Geometry: final body of the model. Coordinates: model frame, mm. Face numbers are marked on the shaded views. A direction names the side the tool comes from. Coordinates: 2 decimals unless noted, no trailing zeros. Order: outer loops, then holes, each group sorted by start corner. A loop starts at its lowest first (then second) coordinate and runs counter-clockwise, first axis right, second up. Notation, with made-up numbers: (-34.75, 88.5) -> (5.25, 88.5) arc R22 cw to (5.25, 111.5) -> close; hole circle Ø8 at (37.25, -21.5). An arc over 180 degrees is marked (long way). Use one line per item in the form item = value.
```python
from build123d import *

# Parameters (mm, degrees)
SKIZZE1_W                       = 36
SKIZZE1_H                       = 38
AUFSATZ_LINEAR_AUSTRAGEN2_DEPTH = 40
VERRUNDUNG1_R                   = 1
SCHNITT_LINEAR_AUSTRAGEN1_REACH = 74.681
SKIZZE2_W                       = 30
SKIZZE2_H                       = 30
VERRUNDUNG2_R                   = 6
DURCHGANGSLOCH_F_R_M31_D        = 3.4
DURCHGANGSLOCH_F_R_M31_DEPTH    = 3
DURCHGANGSLOCH_F_R_M31_TIP      = 1.021463052
SKIZZE5_W                       = 2.5
SKIZZE5_H                       = 38
SKIZZE5_W_2                     = 1
AUFSATZ_LINEAR_AUSTRAGEN3_DEPTH = 2
SKIZZE8_W                       = 1
SKIZZE8_H                       = 38
SCHNITT_LINEAR_AUSTRAGEN3_DEPTH = 1
SKIZZE6_W                       = 2.5
SKIZZE6_H                       = 38
SKIZZE6_W_2                     = 1
AUFSATZ_LINEAR_AUSTRAGEN4_DEPTH = 2
SKIZZE9_W                       = 1
SKIZZE9_H                       = 38
SCHNITT_LINEAR_AUSTRAGEN4_DEPTH = 1
VERRUNDUNG3_R                   = 1
VERRUNDUNG4_R                   = 1
SCHNITT_LINEAR_AUSTRAGEN2_REACH = 75.338
VERRUNDUNG9_R                   = 1
VERRUNDUNG10_R                  = 10


with BuildPart() as part:
    # Skizze1 → Aufsatz-Linear austragen2 (new body)
    with BuildSketch(Plane(origin=(0, 0, 0), x_dir=(1, 0, 0), z_dir=(0, 1, 0))):
        with BuildLine():
            Line((20, -21), (20, 21))
            ThreePointArc((20, 21), (19.460793496, 22.319706051), (18.151722222, 22.884241359))
            ThreePointArc((18.151722222, 22.884241359), (7.231561818, 25.331524584), (-1.857986079, 31.859864147))
            Line((-1.857986079, 31.859864147), (-27.041617117, 22.693772058))
            ThreePointArc((-27.041617117, 22.693772058), (-31.15076398, 18.70575902), (-30.908104914, 12.984705575))
            ThreePointArc((-30.908104914, 12.984705575), (-27.294602816, 1.09378988), (-27.822222222, -11.322847799))
            ThreePointArc((-27.822222222, -11.322847799), (-26.22162429, -18.029054702), (-20, -21))
            Line((-20, -21), (20, -21))
        make_face()
        Rectangle(SKIZZE1_W, SKIZZE1_H, mode=Mode.SUBTRACT)
        with BuildLine():
            Line((16, 21), (-20, 21))
            Line((-20, 21), (-20, -18))
            ThreePointArc((-20, -18), (-23.888515181, -16.143159189), (-24.888888889, -11.951779874))
            ThreePointArc((-24.888888889, -11.951779874), (-24.318489531, 1.471612211), (-28.224978285, 14.326656205))
            ThreePointArc((-28.224978285, 14.326656205), (-28.363640609, 17.595829603), (-26.015556687, 19.874694196))
            Line((-26.015556687, 19.874694196), (-1.583548546, 28.767217922))
            ThreePointArc((-1.583548546, 28.767217922), (6.56927519, 23.437142814), (16, 21))
        make_face(mode=Mode.SUBTRACT)
    extrude(amount=AUFSATZ_LINEAR_AUSTRAGEN2_DEPTH)

    # Verrundung1
    verrundung1_edges = [part.edges().sort_by_distance(p)[0] for p in [
        (20, 20, 21),
        (16, 20, -21),
        (-1.583548546, 20, -28.767217922),
        (-20, 20, 18),
        (-20, 20, -21),
    ]]
    fillet(verrundung1_edges, radius=VERRUNDUNG1_R)

    # Skizze2 → Schnitt-Linear austragen1 (cut, up to next)
    with BuildSketch(Plane(origin=(20, 0, 0), x_dir=(0, 0, -1), z_dir=(1, 0, 0)), mode=Mode.PRIVATE) as schnitt_linear_austragen1_sk1:
        with Locations((0, 20)):
            Rectangle(SKIZZE2_W, SKIZZE2_H)
    schnitt_linear_austragen1_tool1 = extrude(schnitt_linear_austragen1_sk1.sketch, amount=-SCHNITT_LINEAR_AUSTRAGEN1_REACH, mode=Mode.PRIVATE) & part.part
    add(schnitt_linear_austragen1_tool1.solids().sort_by_distance((20, 20, 0))[0], mode=Mode.SUBTRACT)

    # Verrundung2
    verrundung2_edges = [part.edges().sort_by_distance(p)[0] for p in [
        (19, 5, 15),
        (19, 35, 15),
        (19, 35, -15),
        (19, 5, -15),
    ]]
    fillet(verrundung2_edges, radius=VERRUNDUNG2_R)

    # Durchgangsloch für M31
    with Locations(Plane(origin=(-10.456906044, 0, -28.730113233), x_dir=(-0.9396926207859081, 0, 0.34202014332566955), z_dir=(-0.34202014332566955, 0, -0.9396926207859082))):
        with Locations((-4.650779494, 37), (15.349220506, 3), (-4.650779494, 3), (15.349220506, 37)):
            Hole(DURCHGANGSLOCH_F_R_M31_D / 2, depth=DURCHGANGSLOCH_F_R_M31_DEPTH)
            with Locations((0, 0, -(DURCHGANGSLOCH_F_R_M31_DEPTH + DURCHGANGSLOCH_F_R_M31_TIP / 2))):  # 118° drill point
                Cone(0, DURCHGANGSLOCH_F_R_M31_D / 2, DURCHGANGSLOCH_F_R_M31_TIP, mode=Mode.SUBTRACT)

    # Skizze5 → Aufsatz-Linear austragen3 (add)
    with BuildSketch(Plane.XZ):
        with Locations((16.75, 0)):
            Rectangle(SKIZZE5_W, SKIZZE5_H)
        with Locations((-17.5, 0)):
            Rectangle(SKIZZE5_W_2, SKIZZE5_H)
    extrude(amount=-AUFSATZ_LINEAR_AUSTRAGEN3_DEPTH)

    # Skizze8 → Schnitt-Linear austragen3 (cut)
    with BuildSketch(Plane(origin=(0, 2, 0), x_dir=(1, 0, 0), z_dir=(0, 1, 0))):
        with Locations((-17.5, 0)):
            Rectangle(SKIZZE8_W, SKIZZE8_H)
    extrude(amount=-SCHNITT_LINEAR_AUSTRAGEN3_DEPTH, mode=Mode.SUBTRACT)

    # Skizze6 → Aufsatz-Linear austragen4 (add)
    with BuildSketch(Plane(origin=(0, 40, 0), x_dir=(1, 0, 0), z_dir=(0, 1, 0))):
        with Locations((16.75, 0)):
            Rectangle(SKIZZE6_W, SKIZZE6_H)
        with Locations((-17.5, 0)):
            Rectangle(SKIZZE6_W_2, SKIZZE6_H)
    extrude(amount=-AUFSATZ_LINEAR_AUSTRAGEN4_DEPTH)

    # Skizze9 → Schnitt-Linear austragen4 (cut)
    with BuildSketch(Plane.XZ.offset(-38)):
        with Locations((-17.5, 0)):
            Rectangle(SKIZZE9_W, SKIZZE9_H)
    extrude(amount=-SCHNITT_LINEAR_AUSTRAGEN4_DEPTH, mode=Mode.SUBTRACT)

    # Verrundung3
    verrundung3_edges = [part.edges().sort_by_distance(p)[0] for p in [
        (16.75, 2, 19),
        (18, 2, 0),
        (16.75, 2, -19),
        (-17.5, 1, 19),
        (-18, 1, 0),
        (-17.5, 1, -19),
        (18, 20, -19),
        (18, 20, 19),
        (16.75, 38, -19),
        (18, 38, 0),
        (16.75, 38, 19),
        (-18, 20, -19),
        (-18, 20, 19),
        (-17.5, 39, -19),
        (-18, 39, 0),
        (-17.5, 39, 19),
    ]]
    fillet(verrundung3_edges, radius=VERRUNDUNG3_R - 0.0001)  # a hair under: the kernel refuses the full size

    # Verrundung4
    verrundung4_edges = [part.edges().sort_by_distance(p)[0] for p in [
        (-1.857986079, 20, -31.859864147),
    ]]
    fillet(verrundung4_edges, radius=VERRUNDUNG4_R)

    # Skizze7 → Schnitt-Linear austragen2 (cut, up to next)
    with BuildSketch(Plane.XY.offset(21), mode=Mode.PRIVATE) as schnitt_linear_austragen2_sk1:
        with BuildLine():
            Line((-13, 10), (-6.5, 10))
            Line((-6.5, 10), (2.63884007, 14.059753954))
            ThreePointArc((2.63884007, 14.059753954), (6.5, 20), (2.63884007, 25.940246046))
            Line((2.63884007, 25.940246046), (-6.5, 30))
            Line((-6.5, 30), (-13, 30))
            Line((-13, 30), (-13, 10))
        make_face()
    schnitt_linear_austragen2_tool1 = extrude(schnitt_linear_austragen2_sk1.sketch, amount=-SCHNITT_LINEAR_AUSTRAGEN2_REACH, mode=Mode.PRIVATE) & part.part
    add(schnitt_linear_austragen2_tool1.solids().sort_by_distance((-4.747297, 20, 21))[0], mode=Mode.SUBTRACT)

    # Verrundung9
    verrundung9_edges = [part.edges().sort_by_distance(p)[0] for p in [
        (-13, 10, 20),
        (-13, 30, 20),
    ]]
    fillet(verrundung9_edges, radius=VERRUNDUNG9_R)

    # Verrundung10
    verrundung10_edges = [part.edges().sort_by_distance(p)[0] for p in [
        (-6.5, 30, 20),
        (-6.5, 10, 20),
    ]]
    fillet(verrundung10_edges, radius=VERRUNDUNG10_R)


solid = part.part
```
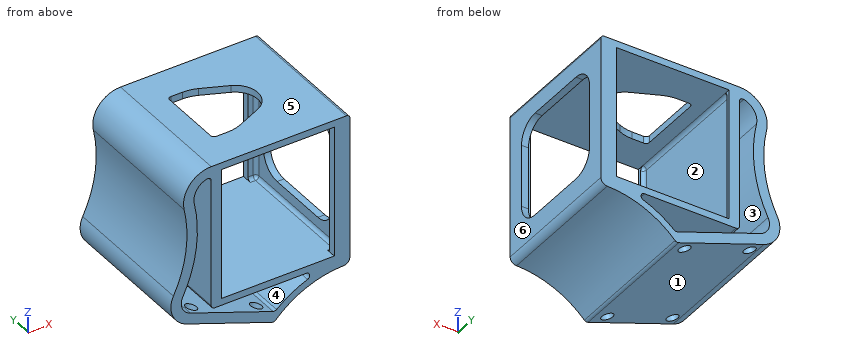
1) Access query for the marked faces 1, 2 and 3. Directions: +Z, -Z, +X, -X, +Y, -Y. A direction counts if a zero-diameter tool reaches every point of the face in a straight line with its end or side. Return the directions, or none.
Results found:
face_1 = -Z, -X, +Y, -Y
face_2 = none
face_3 = +Y, -Y
2) Contact query for flat-ended pins moving along their axis: P1, Ø18.5, axis at y = 29.5, z = 5.5, coming from the -X side; P2, Ø1.5, axis at x = 5.5, y = 23.5, coming from the -Z side; P3, Ø12, axis at y = 10, z = -6.5, coming from the -X side. Output: stop coordinate, or through.
Results found:
P1 = -28
P2 = -26.6
P3 = -30.67
3) Section A-A, the plane z = -12. Give the number of separate pieces and of enclosed holes in the cut face, and give its area (3 significant figures).
Results found:
separate_pieces = 4
enclosed_holes = 0
area = 247 mm2
4) Section B-B, the plane x = 0. Output: boundary loops of the cut face in (y, z), and give its area (3 significant figures).
Results found:
outline = (0, -30.03) -> (40, -30.03) -> (40, -27.41) -> (0, -27.41) -> close; (0, -21) -> (40, -21) -> (40, -19) -> (0, -19) -> close; (0, 19) -> (12.89, 19) -> (12.89, 21) -> (0, 21) -> close; (27.11, 19) -> (40, 19) -> (40, 21) -> (27.11, 21) -> close
area = 236 mm2
5) Material intervals for probe 1 along X at (y, z) = (6.5, -15); probe 2 along Y at (x, z) = (-23, -22.5); probe 3 along Z at (x, y) = (-6, 33), sorted ascending. Write a range as from..to.
Results found:
probe_1 = -31.56..-28.49, -20..-18, 18..20
probe_2 = 0..2.08, 3.92..36.08, 37.92..40
probe_3 = -30.35..-27.16, -21..-19, 19..21
6) Pull-direction query (X, two-part tool) for the marked faces 4, 5 and 6; classes: released by +X, released by -X, zero draft, split by the parting line, or undercut.
Results found:
face_4 = undercut
face_5 = zero draft
face_6 = released by +X
